from build123d import *

# Parameters (mm, degrees)
F1_DEPTH    = 580
F2_SIZE2    = 10
F2_SIZE     = 10
F3_T1_DEPTH = 605
F4_R        = 5
F5_DEPTH    = 28.0010001


# Not quite as in the source:
# - a fillet or chamfer that OpenCascade refuses, or shapes differently, is made with other operations: its cross-section is extruded or revolved along the edge and cut away or added


with BuildPart() as f1:
    # F0 (on Front) → F1 (new body)
    with BuildSketch(Plane.XZ):
        Polygon((30, -14), (30, 14), (-30, 14), (-30, -14), (-15, -14), (-15, -6), (1, -6), (1, -14), align=None)
    extrude(amount=F1_DEPTH)

    # F2
    f2_edges = [f1.edges().sort_by_distance(p)[0] for p in [
        (30, -290, -14),
    ]]
    chamfer(f2_edges, length=F2_SIZE, length2=F2_SIZE2)

    # F3: fillet of radius 5 on 1 edges, made by hand

    # F3_s2 → F3_t1 (cut)
    with BuildSketch(Plane.XZ.offset(-12.5)):
        with BuildLine():
            add(Edge.make_bspline(
                [(30, 9), (30, 14), (25, 14)],
                knots=[0, 0, 0, 1, 1, 1], degree=2, weights=[1, 1, 1]))
            Line((25, 14), (30, 14))
            Line((30, 14), (30, 9))
        make_face()
    extrude(amount=F3_T1_DEPTH, mode=Mode.SUBTRACT)

    # F4 (on face) → F5 (cut, through all)
    with BuildSketch(Plane.XY.offset(14)):
        with Locations((-7, -25)):
            Circle(F4_R)
        with Locations((-7, -290)):
            Circle(F4_R)
        with Locations((-7, -157.5)):
            Circle(F4_R)
        with Locations((-7, -422.5)):
            Circle(F4_R)
        with Locations((-7, -555)):
            Circle(F4_R)
    extrude(amount=-F5_DEPTH, mode=Mode.SUBTRACT)


solid = f1.part
The listing builds one solid part. Answer for the finished solid, in the listing's coordinates (mm). A direction names the side the tool comes from. Give positions to 0.01 mm unless a question says otherwise; leave off trailing zeros. Order: outer loops, then holes, each group sorted by start corner. A loop starts at its lowest first (then second) coordinate and runs counter-clockwise, first axis right, second up. Notation, with made-up numbers: (-3, -9.5) -> (36, -9.5) arc R22 ccw to (36, 11.5) -> close; hole circle Ø9 at (-24, 51). An arc over 180 degrees is marked (long way). Put each result on its own line as item: value.
Item 1: A cutting plane is placed at A-A on x = -7. Give the vertices of the cut face in (y, z), plus the area to 3 significant figures.
Established:
outline: (-580, -6) -> (-560, -6) -> (-560, 14) -> (-580, 14) -> close; (-550, -6) -> (-427.5, -6) -> (-427.5, 14) -> (-550, 14) -> close; (-417.5, -6) -> (-295, -6) -> (-295, 14) -> (-417.5, 14) -> close; (-285, -6) -> (-162.5, -6) -> (-162.5, 14) -> (-285, 14) -> close; (-152.5, -6) -> (-30, -6) -> (-30, 14) -> (-152.5, 14) -> close; (-20, -6) -> (0, -6) -> (0, 14) -> (-20, 14) -> close
area: 10,600 mm^2
Item 2: Straight lines are drawn through the part: line 1 (Y direction, x = -7, z = 1); line 2 (X direction, y = -555, z = 7.75); line 3 (X direction, y = -446, z = -9). For each, find the intervals that lie inside material, in ascending order.
Established:
line 1: y = -580 to -560, -550 to -427.5, -417.5 to -295, -285 to -162.5, -152.5 to -30, -20 to 0
line 2: x = -30 to -12, -2 to 30
line 3: x = -30 to -15, 1 to 25
Item 3: For faces 5 (the face through (-11, -286, -6)), 6 (the face through (-23, -286, -14)), determine the directions among +Z, -Z, +X, -X, +Y, -Y from which every point of the face is accessible in a straight line to the end or side of a thin tool.
Established:
face 5: -Z, +Y, -Y
face 6: -Z, +X, -X, +Y, -Y
Item 4: Given P1, Ø1, axis at x = -0.5, y = -116, coming from the -Z side; P2, Ø6, axis at x = 23, z = -11, coming from the +Y side; P3, Ø9, axis at y = -162, z = -11.5, coming from the +X side, each flat-ended and moving along its own axis, determine where each tip first touches the part or whether it passes through.
Established:
P1: stops at z = -6
P2: stops at y = 0
P3: stops at x = 27
Item 5: For a pull along Y with two mould halves and no side action, classify faces 1 (the face through (0, -580, 0)), 2 (the face through (-7.651, -417.543, 4.14)), 3 (the face through (-7.651, -285.043, 4.14)), 4 (the face through (30, -286, 2)) as released by +Y, released by -Y, zero draft, split by the parting line, or undercut.
Established:
face 1: released by -Y
face 2: undercut
face 3: undercut
face 4: zero draft
